Autodesk Inventor part; units mm, degrees
ref_plane "YZ Plane" through (0, 0, 0) normal (1, 0, 0) x (0, 1, 0)
ref_plane "XZ Plane" through (0, 0, 0) normal (0, 1, 0) x (-1, 0, 0)
ref_plane "XY Plane" through (0, 0, 0) normal (0, 0, 1) x (1, 0, 0)
sketch "Sketch1" plane through (0, 0, 0) normal (0, 1, 0) x (-1, 0, 0)
  line L0 (0, 0) -> (38.1, 0)
  line L1 (38.1, 0) -> (38.1, -241.3)
  line L2 (38.1, -241.3) -> (0, -241.3)
  line L3 (0, -241.3) -> (0, 0)
  dimension "d0" = 38.1
  dimension "d1" = 241.3
extrude "Extrusion1" add sketch "Sketch1" along normal blind 31.75
sketch "Sketch2" plane through (0, 0, 0) normal (1, 0, 0) x (0, 0, -1)
  line L0 (241.3, 0) -> (0, 0)
  line L1 (120.65, 0) -> (120.65, 22.86)
  line L2 (120.65, 22.86) -> (212.09, 22.86)
  line L3 (241.3, 31.75) -> (0, 31.75)
  line L4 (120.65, 22.86) -> (29.21, 22.86)
  line L5 (29.21, 22.86) -> (29.21, 0)
  line L6 (212.09, 22.86) -> (212.09, 0)
  line L7 (212.09, 0) -> (29.21, 0)
  dimension "d4" = 22.86
  dimension "d5" = 91.44
  dimension "d7" = 91.44
extrude "Extrusion2" cut sketch "Sketch2" against normal through all
fillet "Fillet1" radius 1.27 2 edges at (-19.05, 22.86, -212.09) (-19.05, 22.86, -29.21)
sketch "Sketch5" plane through (0, 0, -241.3) normal (1, 0, 0) x (0, 0, -1)
  line L0 (0, 31.75) -> (-22.225, 31.75)
  line L1 (-22.225, 31.75) -> (-22.225, 19.05)
  line L2 (-22.225, 19.05) -> (0, 19.05)
  line L3 (0, 19.05) -> (0, 31.75)
  line L4 (-241.3, 0) -> (-241.3, 31.75)
  line L5 (-241.3, 31.75) -> (-219.075, 31.75)
  line L6 (-219.075, 31.75) -> (-219.075, 19.05)
  line L7 (-219.075, 19.05) -> (-241.3, 19.05)
  line L8 (-241.3, 19.05) -> (-241.3, 31.75)
  dimension "d29" = 22.225
  dimension "d30" = 12.7
  dimension "d31" = 22.225
  dimension "d32" = 12.7
extrude "Extrusion3" cut sketch "Sketch5" against normal through all
fillet "Fillet2" radius 3.175 4 edges at (-19.05, 19.05, -219.075) (-19.05, 31.75, -219.075) (-19.05, 31.75, -22.225) (-19.05, 19.05, -22.225)
sketch "Sketch6" plane through (-38.1, 19.05, -241.3) normal (0, 1, 0) x (1, 0, 0)
  line L0 (0, 0) -> (38.1, 0)
  line L1 (38.1, 0) -> (38.1, -19.05)
  point P0 (38.1, -241.3)
  point P1 (19.05, -12.7)
  dimension "d36" = 12.7
  dimension "d44" = 19.05
hole "Hole3" at (-19.05, 19.05, -228.6) direction (0, -1, 0) diameter 5.1594 end through all counterbore diameter 12.7 counterbore depth 1.5875
sketch "Sketch7" plane through (-38.1, 19.05, 0) normal (0, 1, 0) x (1, 0, 0)
  line L0 (38.1, 0) -> (0, 0)
  line L1 (38.1, 19.05) -> (38.1, 0)
  point P0 (19.05, 12.7)
  dimension "d45" = 12.7
  dimension "d46" = 19.05
hole "Hole4" at (-19.05, 19.05, -12.7) direction (0, -1, 0) diameter 5.1594 end through all counterbore diameter 12.7 counterbore depth 1.5875
fillet "Fillet3" radius 3.175 4 edges at (0, 9.525, 0) (-38.1, 9.525, 0) (0, 9.525, -241.3) (-38.1, 9.525, -241.3)
sketch "Sketch11" plane through (0, 0, 0) normal (0, -1, 0) x (1, 0, 0)
  circle A0 centre (-19.05, -228.6) radius 2.5797
  point P0 (0, 0)
hole "Hole5" at (-19.05, 0, -228.6) direction (0, 1, 0) diameter 11.43 depth 6.35 tip angle 118
sketch "Sketch12" plane through (0, 0, 0) normal (0, -1, 0) x (1, 0, 0)
  circle A0 centre (-19.05, -12.7) radius 2.5797
  point P0 (0, 0)
hole "Hole6" at (-19.05, 0, -12.7) direction (0, 1, 0) diameter 11.43 depth 6.35 tip angle 118
properties part number "Battery Strap"
Build history of the part. All positions in model axes, mm. A direction names the side the tool comes from. Give positions to 0.01 mm unless a question says otherwise; leave off trailing zeros. Write each loop counter-clockwise with the first axis right and the second up, starting at its lowest first coordinate (ties: lowest second). Pieces come first, ordered by that corner, then holes. Notation, with made-up numbers: (-35.75, -10.5) - (10.25, -10.5) arc R15 cw to (10.25, 17.5) - close; hole circle Ø10 at (-22.5, 71.25). An arc over 180 degrees is marked (long way). Use one line per item in the form item = value. Start each with the question number.
1. Drop flat-ended pins along their axis: pin 1 Ø1.9 at (x, y) = (-21.5, 26) entering from +Z (3 decimals); pin 2 Ø14.5 at (x, z) = (-19.05, -12.7) entering from +Y; pin 3 Ø6 at (x, y) = (-9, 22.5) entering from -Z; pin 4 Ø10 at (y, z) = (27.5, -123.5) entering from +X. Give the stop position or say it passes through.
2. 3-axis set-ups, long thin cutter, end or side, ignore diameter. For faces 1 (the face through (-19.3, 3.22, -222.89)), 2 (the face through (-24.404, 18.245, -9.286)), 3 (the face through (-19, 11, -212.09)), 4 (the face through (-19, 25, -22.225)): which of +Z, -Z, +X, -X, +Y, -Y reach the whole face in a straight line?
3. Band-saw the part on C-C on z = -145. Write the cut outline in (x, y).
4. Two-plate mould, pull along Z, no slides. Class faces 5 (the face through (-19, 9, -241.3)), 6 (the face through (-19, 19.05, -236)), 7 (the face through (-19, 22.86, -119)): released by +Z, released by -Z, zero draft, split by the parting line, or undercut.
5. Band-saw the part on B-B on x = -31. Write the cut outline in (y, z) (3 decimals).
6. Probe line 1 (Z direction, x = -19.05, y = 4.75) (3 decimals); line 2 (Z direction, x = -3, y = 11); line 3 (X direction, y = 2.5, z = -228.6) (3 decimals). List the from-to ranges inside material, lowest first. Write a range as [from, to].
Conclusion:
q1.pin_1 = -22.225
q1.pin_2 = 19.18
q1.pin_3 = -220.62
q1.pin_4 = 0
q2.face_1 = -Y
q2.face_2 = +Y
q2.face_3 = +X, -X, -Y
q2.face_4 = +Z, +X, -X, +Y
q3.outline = (-38.1, 22.86) - (0, 22.86) - (0, 31.75) - (-38.1, 31.75) - close
q4.face_5 = released by -Z
q4.face_6 = zero draft
q4.face_7 = undercut
q5.outline = (0, -241.3) - (19.05, -241.3) - (19.05, -222.25) arc R3.175 cw to (22.225, -219.075) - (28.575, -219.075) arc R3.175 ccw to (31.75, -215.9) - (31.75, -25.4) arc R3.175 ccw to (28.575, -22.225) - (22.225, -22.225) arc R3.175 cw to (19.05, -19.05) - (19.05, 0) - (0, 0) - (0, -29.21) - (21.59, -29.21) arc R1.27 cw to (22.86, -30.48) - (22.86, -210.82) arc R1.27 cw to (21.59, -212.09) - (0, -212.09) - close
q6.line_1 = [-241.3, -234.315], [-222.885, -212.09], [-29.21, -18.415], [-6.985, 0]
q6.line_2 = [-241.3, -212.09], [-29.21, 0]
q6.line_3 = [-38.1, -24.765], [-13.335, 0]
